The listing builds one solid part. Answer for the finished solid, in the listing's coordinates (mm). A direction names the side the tool comes from. Coordinates: 2 decimals unless noted, no trailing zeros. Order: outer loops, then holes, each group sorted by start corner. A loop starts at its lowest first (then second) coordinate and runs counter-clockwise, first axis right, second up. Notation, with made-up numbers: (53.25, 4.25) - (86.25, 4.25) arc R24 ccw to (86.25, 42.25) - close; hole circle Ø8 at (67, 1). An arc over 180 degrees is marked (long way). Use a Markdown table: item, result. Add a question column.
Item 1: The mould has two halves that part along X. Classify faces 1 (the flat face through (19.05, -47, 6)), 2 (the flat face through (0, -27, 12.7)), 3 (the cylindrical face through (-23.06, -6.44, 54.33)), 4 (the cylindrical face through (22.58, -6.44, 54.81)): released by +X, released by -X, zero draft, split by the parting line, or undercut.
Item 2: The part is cut by section D-D, the plane y = -23.5. Give the vertices of the cut face in (x, z).
Item 3: The part is cut by section B-B, the plane z = 43. Give the vertices of the cut face in (x, y), then the cut area to 3 significant figures.
Item 4: For faces 5 (the flat face through (0, -42.081, 6)), 6 (the flat face through (8, 0, 24)), 7 (the flat face through (0, -12.7, 22)), determine the directions among +Z, -Z, +X, -X, +Y, -Y from which every point of the face is accessible in a straight line to the end or side of a thin tool.
Item 5: The part is cut by section A-A, the plane x = 0. Give the vertices of the cut face in (y, z).
Item 6: Find the intervals of material crossed by line 1 along Z through (x, y) = (0, -5.25); line 2 along Z through (x, y) = (13, -36); line 3 along Y through (x, z) = (11.5, 15.5), in increasing order.
Item 7: Flat-ended cylindrical pins translate along their axes: P1, Ø4, axis at x = -7, z = 4.5, coming from the -Y side; P2, Ø8, axis at x = 12, y = -19, coming from the +Z side; P3, Ø2.5, axis at y = -44.5, z = 4.5, coming from the +X side. Find the tip coordinate at first contact, or state that the pin passes through.
Item 8: The part is cut by section C-C, the plane x = 22. Give the vertices of the cut face in (y, z).
from build123d import *

# Parameters (mm, degrees)
F1_DEPTH = 31.75
F3_DEPTH = 25.4
F4_W     = 38.1
F4_H     = 8.718614
F5_DEPTH = 25.4
F6_R     = 14.857396
F7_DEPTH = 25.4


with BuildPart() as f1:
    # F0 (on Right) → F1 (new body, symmetric)
    with BuildSketch(Plane.YZ):
        Polygon((-50.8, 0), (0, 0), (0, 63.5), (-12.7, 63.5), (-12.7, 12.7), (-50.8, 12.7), align=None)
    extrude(amount=F1_DEPTH, both=True)

    # F2 (on face) → F3 (cut)
    with BuildSketch(Plane.XY.offset(12.7)):
        with BuildLine():
            ThreePointArc((-19.05, -50.8), (-28.030256, -47.080256), (-31.75, -38.1))
            Line((-31.75, -38.1), (-31.75, -50.8))
            Line((-31.75, -50.8), (-19.05, -50.8))
        make_face()
        with BuildLine():
            Line((31.75, -50.8), (31.75, -38.1))
            ThreePointArc((31.75, -38.1), (28.030256, -47.080256), (19.05, -50.8))
            Line((19.05, -50.8), (31.75, -50.8))
        make_face()
    extrude(amount=-F3_DEPTH, mode=Mode.SUBTRACT)

    # F4 (on face) → F5 (cut)
    with BuildSketch(Plane.XY.offset(12.7)):
        with Locations((0, -46.440693)):
            Rectangle(F4_W, F4_H)
    extrude(amount=-F5_DEPTH, mode=Mode.SUBTRACT)

    # F6 (on face) → F7 (cut)
    with BuildSketch(Plane.XZ.offset(12.7)):
        with BuildLine():
            Line((-31.75, 63.5), (-31.75, 33.02))
            ThreePointArc((-31.75, 33.02), (-22.822615, 54.572615), (-1.27, 63.5))
            Line((-1.27, 63.5), (-31.75, 63.5))
        make_face()
        with BuildLine():
            Line((31.75, 63.5), (1.27, 63.5))
            ThreePointArc((1.27, 63.5), (22.822615, 54.572615), (31.75, 33.02))
            Line((31.75, 33.02), (31.75, 63.5))
        make_face()
        with Locations((0, 37.374914)):
            Circle(F6_R)
    extrude(amount=-F7_DEPTH, mode=Mode.SUBTRACT)


solid = f1.part
Solution:
| question | item | result |
|---|---|---|
| 1 | face 1 | undercut |
| 1 | face 2 | zero draft |
| 1 | face 3 | released by -X |
| 1 | face 4 | released by +X |
| 2 | outline | (-31.75, 0) - (31.75, 0) - (31.75, 12.7) - (-31.75, 12.7) - close |
| 3 | outline | (-30.07, -12.7) - (-13.75, -12.7) - (-13.75, 0) - (-30.07, 0) - close; (13.75, -12.7) - (30.07, -12.7) - (30.07, 0) - (13.75, 0) - close |
| 3 | area | 414 mm2 |
| 4 | face 5 | +Z, -Z, -Y |
| 4 | face 6 | +Z, -Z, +X, -X, +Y |
| 4 | face 7 | +Z, +X, -X, -Y |
| 5 | outline | (-42.08, 0) - (0, 0) - (0, 22.52) - (-12.7, 22.52) - (-12.7, 12.7) - (-42.08, 12.7) - close; (-12.7, 52.23) - (0, 52.23) - (0, 63.5) - (-12.7, 63.5) - close |
| 6 | line 1 | z = 0 to 22.52, 52.23 to 63.5 |
| 6 | line 2 | z = 0 to 12.7 |
| 6 | line 3 | y = -12.7 to 0 |
| 7 | P1 | stops at y = -42.08 |
| 7 | P2 | stops at z = 12.7 |
| 7 | P3 | stops at x = 30.66 |
| 8 | outline | (-50.45, 0) - (0, 0) - (0, 55.36) - (-12.7, 55.36) - (-12.7, 12.7) - (-50.45, 12.7) - close |
